Model file for the job. Use its own axes, mm. A direction names the side the tool comes from. Give positions to 0.01 mm unless a question says otherwise; leave off trailing zeros. Loops run counter-clockwise (first coordinate to the right, second up) from the corner with the lowest first, then second, coordinate; pieces in that order, holes last. Notation, with made-up numbers: M 51,54 L 87,54 A21 ccw 87,90 Z; hole C 57,60.5 d7. An arc over 180 degrees is marked long. Answer in a Markdown table with one row per item.
```python
from build123d import *

# Parameters (mm, degrees)
F0_R     = 50.355845
F0_R_2   = 19.23064
F2_DEPTH = 25.4
F3_DEPTH = 159.512
F6_DEPTH = 39.624
F7_DEPTH = 60.452


with BuildPart() as f2:
    # F0 (on Front) → F2 (new body)
    with BuildSketch(Plane.XZ):
        Circle(F0_R)
        Circle(F0_R_2, mode=Mode.SUBTRACT)
    extrude(amount=F2_DEPTH)

    # F1 (on face) → F3 (cut)
    with BuildSketch(Plane.XZ):
        with BuildLine():
            ThreePointArc((-6.010604, 44.439051), (-25.277411, 39.727291), (-36.75336, 23.549741))
            Line((-36.75336, 23.549741), (-23.549741, 16.652327))
            ThreePointArc((-23.549741, 16.652327), (-16.553358, 25.609562), (-6.010604, 29.855948))
            Line((-6.010604, 29.855948), (-6.010604, 44.439051))
        make_face()
    extrude(amount=F3_DEPTH, mode=Mode.SUBTRACT)

    # F4 (on face) → F6 (cut)
    with BuildSketch(Plane.XZ.offset(25.4)):
        with BuildLine():
            ThreePointArc((-17.440604, -23.155604), (-25.338416, -12.904348), (-26.308708, 0))
            Line((-26.308708, 0), (-40.69474, 0))
            ThreePointArc((-40.69474, 0), (-40.96629, -17.711086), (-26.899915, -28.476467))
            Line((-26.899915, -28.476467), (-17.440604, -23.155604))
        make_face()
    extrude(amount=-F6_DEPTH, mode=Mode.SUBTRACT)

    # F5 (on face) → F7 (cut)
    with BuildSketch(Plane.XZ.offset(25.4)):
        with BuildLine():
            Line((15.272845, 37.344571), (11.528536, 22.367328))
            ThreePointArc((11.528536, 22.367328), (22.950874, 19.787073), (30.841293, 11.134396))
            Line((30.841293, 11.134396), (40.300604, 15.864052))
            ThreePointArc((40.300604, 15.864052), (32.595246, 32.2069), (15.272845, 37.344571))
        make_face()
        with BuildLine():
            ThreePointArc((26.702844, -17.440604), (16.707275, -24.978413), (4.631122, -28.279396))
            Line((4.631122, -28.279396), (4.631122, -39.512329))
            ThreePointArc((4.631122, -39.512329), (22.846027, -38.484063), (33.600256, -23.746809))
            Line((33.600256, -23.746809), (26.702844, -17.440604))
        make_face()
    extrude(amount=-F7_DEPTH, mode=Mode.SUBTRACT)


solid = f2.part
```
Q1. 3-axis set-ups, long thin cutter, end or side, ignore diameter. For faces 1 (the face through (22, -25.4, 1)), 2 (the face through (-25.042, -12.522, 39.886)): which of +Z, -Z, +X, -X, +Y, -Y reach the whole face in a straight line?
Reported:
| item | result |
|---|---|
| face 1 | +Z, -Z, +X, -X, -Y |
| face 2 | +Y, -Y |
Q2. Saw through at A-A (x = 0). Give the cut face in (y, z).
Reported:
| item | result |
|---|---|
| outline | M -25.4,-50.36 L 0,-50.36 L 0,-19.23 L -25.4,-19.23 Z; M -25.4,19.23 L 0,19.23 L 0,50.36 L -25.4,50.36 Z |
Q3. Saw through at D-D (x = -30). Give the cut face in (y, z), and give its area (3 significant figures).
Reported:
| item | result |
|---|---|
| outline | M -25.4,-40.44 L 0,-40.44 L 0,-27.62 L -25.4,-27.62 Z; M -25.4,0 L 0,0 L 0,20.02 L -25.4,20.02 Z; M -25.4,35.7 L 0,35.7 L 0,40.44 L -25.4,40.44 Z |
| area | 955 mm² |
Q4. Saw through at B-B (y = -23). Give the cut face in (x, z).
Reported:
| item | result |
|---|---|
| outline | C 0,0 d100.71; hole M -40.69,0 A19.69 ccw -26.9,-28.48 L -17.44,-23.16 A22.57 cw -26.31,0 Z; hole M -36.75,23.55 L -23.55,16.65 A21.91 cw -6.01,29.86 L -6.01,44.44 A28.38 ccw Z; hole C 0,0 d38.46; hole M 4.63,-39.51 A21.33 ccw 33.6,-23.75 L 26.7,-17.44 A33.2 cw 4.63,-28.28 Z; hole M 11.53,22.37 A19.52 cw 30.84,11.13 L 40.3,15.86 A22.11 ccw 15.27,37.34 Z |
Q5. Mould opens along X. For faces 3 (the face through (48.03, -12.52, 15.13)), 4 (the face through (13.427, -12.878, 29.961)), 5 (the face through (22, 0, 1)) say: released by +X, released by -X, zero draft, split by the parting line, or undercut.
Reported:
| item | result |
|---|---|
| face 3 | split by the parting line |
| face 4 | undercut |
| face 5 | zero draft |
Q6. Probe probe 1 along Z at (x, y) = (0, -7.5); probe 2 along X at (y, z) = (-13.75, 16); probe 3 along X at (y, z) = (-21, -3.5). List the from-to ranges inside material, lowest first.
Reported:
| item | result |
|---|---|
| probe 1 | -50.36 to -19.23, 19.23 to 50.36 |
| probe 2 | -47.75 to -10.67, 10.67 to 27.62, 40.3 to 47.75 |
| probe 3 | -50.23 to -42.12, -26.79 to -18.91, 18.91 to 50.23 |
Q7. Drop flat-ended pins along their axis: pin 1 (4.5 mm diameter, centred on x = -33, y = -11, fed in from -Z); pin 2 (5 mm diameter, centred on y = -10.5, z = 33.5, fed in from -X); pin 3 (10 mm diameter, centred on x = 2, z = 9.5, fed in from -Y); pin 4 (10 mm diameter, centred on y = -16.5, z = -28, fed in from -X). Give the stop position or say it passes through.
Reported:
| item | result |
|---|---|
| pin 1 | z = -39.88 |
| pin 2 | x = -39.68 |
| pin 3 | through |
| pin 4 | x = -44.8 |
Q8. Saw through at C-C (z = 2). Give the cut face in (x, y), and give its area (3 significant figures).
Reported:
| item | result |
|---|---|
| outline | M -50.32,-25.4 L -19.13,-25.4 L -19.13,0 L -50.32,0 Z; M 19.13,-25.4 L 50.32,-25.4 L 50.32,0 L 19.13,0 Z |
| area | 1,580 mm² |
